Check sheet for the drawn part. Datum: minimum x, y, z corner. Units: mm. Round coordinates to 2 decimals unless told otherwise and drop trailing zeros. Write each loop counter-clockwise with the first axis right and the second up, starting at its lowest first coordinate (ties: lowest second). Pieces come first, ordered by that corner, then holes. Notation, with made-up numbers: M -16.75,-30 L 18.25,-30 A15 cw 18.25,-17 Z; hole C 84,71.5 d6. An arc over 180 degrees is marked long. Use a Markdown table: item, result.
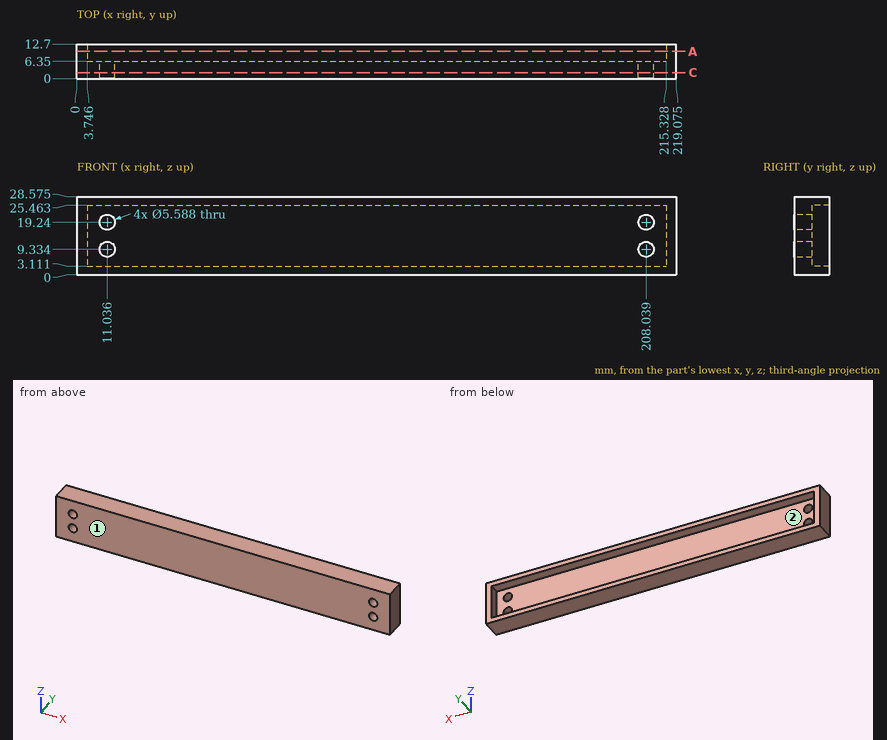
Item 1: Material ranges on line 1 along X through (y, z) = (3, 9) (1 decimal); line 2 along Z through (x, y) = (24, 11.5) (1 decimal); line 3 along X through (y, z) = (7, 23.5) (1 decimal), recorded low to high. Write a range as from..to.
Outcome:
| item | result |
|---|---|
| line 1 | x = 0..8.3, 13.8..205.3, 210.8..219.1 |
| line 2 | z = 0..3.1, 25.5..28.6 |
| line 3 | x = 0..3.7, 215.3..219.1 |
Item 2: Mould release check, pull along Z, two halves, no side actions. Record for the marked faces 1 and 2: +Z half, -Z half, draft (parallel to the pull), parting line (faces both ways), or undercut.
Outcome:
| item | result |
|---|---|
| face 1 | draft |
| face 2 | undercut |
Item 3: Cross-section at A-A, the plane y = 10. Record the cut outline in (x, z) (1 decimal), and give its area (3 significant figures).
Outcome:
| item | result |
|---|---|
| outline | M 0,0 L 219.1,0 L 219.1,28.6 L 0,28.6 Z; hole M 3.7,3.1 L 215.3,3.1 L 215.3,25.5 L 3.7,25.5 Z |
| area | 1,530 mm2 |
Item 4: Cross-section at C-C, the plane y = 2.25. Record the cut outline in (x, z) (1 decimal).
Outcome:
| item | result |
|---|---|
| outline | M 0,0 L 219.1,0 L 219.1,28.6 L 0,28.6 Z; hole C 11,9.3 d5.6; hole C 11,19.2 d5.6; hole C 208,9.3 d5.6; hole C 208,19.2 d5.6 |
Item 5: Go/stop test with flat-tipped pins: pin 1 (9 mm diameter, centred on x = 208.04, z = 19.24, fed in from +Y); pin 2 (5 mm diameter, centred on x = 208.04, z = 9.33, fed in from +Y). Record where each tip stops, or that it passes through.
Outcome:
| item | result |
|---|---|
| pin 1 | stops at y = 6.35 |
| pin 2 | passes through |
